Here's how the part is built. I have some questions about the finished solid (model axes, mm). A direction names the side the tool comes from. Give positions to 0.01 mm unless a question says otherwise; leave off trailing zeros. Order: outer loops, then holes, each group sorted by start corner. A loop starts at its lowest first (then second) coordinate and runs counter-clockwise, first axis right, second up.
Autodesk Inventor part; units mm, degrees
ref_plane "YZ Plane" through (0, 0, 0) normal (1, 0, 0) x (0, 1, 0)
ref_plane "XZ Plane" through (0, 0, 0) normal (0, 1, 0) x (-1, 0, 0)
ref_plane "XY Plane" through (0, 0, 0) normal (0, 0, 1) x (1, 0, 0)
sketch "Sketch1" plane through (0, 0, 0) normal (0, 0, 1) x (1, 0, 0)
  line L0 (-490, 52) -> (490, 52)
  line L1 (490, 52) -> (490, 0)
  line L2 (490, 0) -> (-490, 0)
  line L3 (-490, 0) -> (-490, 52)
  point P0 (0, 0)
  point P1 (0, 0)
  dimension "d0" = 980
  dimension "d1" = 52
extrude "Plate1" add sketch "Sketch1" along normal blind 2
sketch "Sketch2" plane through (490, 2, 0) normal (0, -1, 0) x (1, 0, 0)
  line L0 (-980, 0) -> (0, 0)
  line L1 (0, 0) -> (0, 20)
  line L2 (0, 20) -> (-980, 20)
  line L3 (-980, 20) -> (-980, 0)
edge flange "Flange1" height 20 angle 90 thickness 2 bend radius 2.75 thickness toward (0, -1, 0) relief round relief width 2 relief depth 1 edges at (0, 0, 2) wall of the first edge with corners at (-490, 2, 0) (490, 2, 0) (490, 2, 20) (-490, 2, 20)
bend "Bend1"
corner "Corner1"
sketch "Sketch11" plane through (0, 0, 0) normal (0, 0, 1) x (1, 0, 0)
  line L0 (-490, 52) -> (490, 52)
  circle A0 centre (0, 52) radius 30
  line L1 (-490, 0) -> (490, 0)
  line L2 (246.05, 0) -> (243.95, 0)
  line L3 (243.95, 0) -> (243.95, 27)
  line L4 (243.95, 27) -> (246.05, 27)
  line L5 (246.05, 27) -> (246.05, 0)
  line L6 (-243.95, 0) -> (-246.05, 0)
  line L7 (-246.05, 0) -> (-246.05, 27)
  line L8 (-246.05, 27) -> (-243.95, 27)
  line L9 (-243.95, 27) -> (-243.95, 0)
  line L10 (0, 52) -> (0, 0) construction
  line L11 (246.05, 27) -> (246.05, 52)
  line L12 (243.95, 27) -> (243.95, 52)
  line L13 (-243.95, 27) -> (-243.95, 52)
  line L14 (-246.05, 27) -> (-246.05, 52)
  point P0 (30, 52)
  point P1 (-30, 52)
  point P2 (-245, 27)
  point P3 (245, 27)
  dimension "d44" = 60
  dimension "d47" = 2.1
  dimension "d49" = 490
  dimension "d50" = 27
extrude "Extrusion4" cut sketch "Sketch11" along normal through all both and the other way through all contours L0 L13 L8 L14 | L0 A0 | L0 L11 L4 L12 picked at (3.546, 42.6498)
sketch "Sketch9" plane through (0, 0, 2) normal (0, 0, 1) x (1, 0, 0)
  line L0 (475.4727, 47) -> (475.4727, 35) construction
  line L1 (475.4727, 35) -> (275.4727, 35) construction
  line L2 (275.4727, 35) -> (275.4727, 47) construction
  line L3 (275.4727, 47) -> (475.4727, 47) construction
  line L4 (-490, 52) -> (490, 52)
  point P0 (0, 0)
  point P1 (1, 52)
  dimension "d38" = 200
  dimension "d39" = 12
  dimension "d43" = 5
mark "Mark3"
equation "\"d1\" = СПИНА_Стрингер_1_высота"
equation "\"d43\" = d42"
equation "\"d2\" = Thickness"
equation "\"d3\" = BendReliefWidth"
equation "\"d4\" = BendReliefDepth"
equation "\"d5\" = MinimumRemnant"
equation "\"d6\" = TransitionRadius"
equation "\"d9\" = BendRadius"
equation "\"d10\" = CornerReliefSize"
equation "\"d11\" = GapSize"
equation "\"d12\" = JacobiRadiusSize"
equation "\"BendReliefWidth\" = Thickness"
equation "\"BendReliefDepth\" = 0.5 * Thickness"
equation "\"CornerReliefSize\" = 4 * Thickness"
equation "\"MinimumRemnant\" = 2 * Thickness"
equation "\"TransitionRadius\" = BendRadius"
equation "\"JacobiRadiusSize\" = BendRadius"
equation "\"GapSize\" = Thickness"
properties part number "MSC 205 STRINGER BACK ^" material "Stainless Steel"
Q1. If we section it at B-B on z = 13.5: List the corners of the cut face in (x, y) for me, plus the area to 3 significant figures.
Filled sheet:
outline: (-490, 0) - (490, 0) - (490, 2) - (-490, 2) - close
area: 1,960 mm2
Q2. For faces 1 (the face through (-490, 20, 1)), 2 (the face through (7, 2, 12)), which set-ups out of +Z, -Z, +X, -X, +Y, -Y let a thin tool reach every point of the face, with its end or its side?
Filled sheet:
face 1: +Z, -Z, -X, +Y, -Y
face 2: +Z, +X, -X, +Y
Q3. If we section it at C-C on x = -367.5: List the corners of the cut face in (y, z) for me, plus the area to 3 significant figures.
Filled sheet:
outline: (0, 4.75) arc R4.75 ccw to (4.75, 0) - (52, 0) - (52, 2) - (4.75, 2) arc R2.75 cw to (2, 4.75) - (2, 20) - (0, 20) - close
area: 137 mm2
Q4. If we section it at A-A on x = 0: List the corners of the cut face in (y, z) for me.
Filled sheet:
outline: (0, 4.75) arc R4.75 ccw to (4.75, 0) - (22, 0) - (22, 2) - (4.75, 2) arc R2.75 cw to (2, 4.75) - (2, 20) - (0, 20) - close
Q5. Thinking about a two-plate mould opening in X: for faces 3 (the face through (-7, 18, 2)), 4 (the face through (0.66, 22.007, 0.986)), 5 (the face through (490, 20, 1)), which applies, released by +X, released by -X, zero draft, split by the parting line, or undercut?
Filled sheet:
face 3: zero draft
face 4: undercut
face 5: released by +X
Q6. I need wall thicknesses on L1, parallel to Z at x = 282, y = 31; L2, parallel to Y at x = 79, z = 2.5. Which ranges of each line are inside material? Lowest first, please.
Filled sheet:
L1: z = 0 to 2
L2: y = 0.57 to 3.17
Q7. I'm going to push flat-ended pins straight in: P1, Ø1, axis at x = -245.5, z = 0.5, coming from the +Y side; P2, Ø7.5, axis at x = -25.5, z = 13.5, coming from the +Y side; P3, Ø1, axis at x = -291.5, y = 29.5, coming from the +Z side; P4, Ø2, axis at y = 8.5, z = 3.5, coming from the +X side. Where does each tip first touch, or does it pass through?
Filled sheet:
P1: stops at y = 27
P2: stops at y = 2
P3: stops at z = 2
P4: passes through
